```python
from build123d import *

# Parameters (mm, degrees)
SKETCH1_R           = 177.8
BOSS_EXTRUDE1_DEPTH = 12.7
SKETCH2_R           = 12.7
BOSS_EXTRUDE2_DEPTH = 101.6


with BuildPart() as part:
    # Sketch1 → Boss-Extrude1 (new body, symmetric)
    with BuildSketch(Plane(origin=(0, 0, 0), x_dir=(1, 0, 0), z_dir=(0, 1, 0))):
        Circle(SKETCH1_R)
    extrude(amount=BOSS_EXTRUDE1_DEPTH, both=True)

    # Sketch2 → Boss-Extrude2 (add)
    with BuildSketch(Plane(origin=(0, 12.7, 0), x_dir=(1, 0, 0), z_dir=(0, 1, 0))):
        with Locations((0, 88.9)):
            Circle(SKETCH2_R)
        with Locations((0, -88.9)):
            Circle(SKETCH2_R)
        with Locations((88.9, 0)):
            Circle(SKETCH2_R)
        with Locations((-88.9, 0)):
            Circle(SKETCH2_R)
    extrude(amount=BOSS_EXTRUDE2_DEPTH)


solid = part.part
```
Geometry check sheet. Reference: the model listing, model coordinates, mm. A direction names the side the tool comes from. Coordinates: 2 decimals unless noted, no trailing zeros. Loops run counter-clockwise (first coordinate to the right, second up) from the corner with the lowest first, then second, coordinate; pieces in that order, holes last. Notation, with made-up numbers: (39.5, 88) - (84.5, 88) arc R13 ccw to (84.5, 103) - close; hole circle Ø10 at (73.25, -38). An arc over 180 degrees is marked (long way). One line per item, written item: value. Start each with the question number.
(1) Depth check by flat-ended pin: P1, Ø5, axis at x = -99, z = -65, coming from the +Y side; P2, Ø10, axis at y = 79, z = 4, coming from the -X side. Enter the tip coordinate at first touch or a pass-through.
(2) Cross-section at C-C on x = -88.9. Enter the section's corners in (y, z).
(3) Cross-section at B-B on y = 42. Enter the section's corners in (x, z).
(4) Material ranges on line 1 (Y direction, x = -51.5, z = 98.5); line 2 (Z direction, x = 11.5, y = 30.5); line 3 (X direction, y = -0.5, z = -37), recorded low to high. Write a range as [from, to].
(5) Tool access check on faces 4 (the cylindrical face through (169.59, 0.18, -53.41)), 5 (the cylindrical face through (-1.653, 62.789, 76.308)). Record the directions out of +Z, -Z, +X, -X, +Y, -Y that give a thin tool (end or side, any length) a straight path to the whole face; none if there is none.
(6) Cross-section at A-A on z = 0. Enter the section's corners in (x, y), plus the area to 3 significant figures.
(7) Cross-section at D-D on y = 0. Enter the section's corners in (x, z).
(8) Mould release check, pull along Z, two halves, no side actions. Record for faces 1 (the cylindrical face through (101.014, 62.789, -3.815)), 2 (the cylindrical face through (-1.653, 62.789, -101.492)), 3 (the flat face through (0, 114.3, -89)): released by +Z, released by -Z, zero draft, split by the parting line, or undercut.
Results below:
1. P1: stops at y = 12.7
1. P2: stops at x = -101.6
2. outline: (-12.7, -153.98) - (12.7, -153.98) - (12.7, -12.7) - (114.3, -12.7) - (114.3, 12.7) - (12.7, 12.7) - (12.7, 153.98) - (-12.7, 153.98) - close
3. outline: circle Ø25.4 at (-88.9, 0); circle Ø25.4 at (0, -88.9); circle Ø25.4 at (0, 88.9); circle Ø25.4 at (88.9, 0)
4. line 1: y = [-12.7, 12.7]
4. line 2: z = [-94.29, -83.51], [83.51, 94.29]
4. line 3: x = [-173.91, 173.91]
5. face 4: +Y, -Y
5. face 5: +Y
6. outline: (-177.8, -12.7) - (177.8, -12.7) - (177.8, 12.7) - (101.6, 12.7) - (101.6, 114.3) - (76.2, 114.3) - (76.2, 12.7) - (-76.2, 12.7) - (-76.2, 114.3) - (-101.6, 114.3) - (-101.6, 12.7) - (-177.8, 12.7) - close
6. area: 14,200 mm2
7. outline: circle Ø355.6 at (0, 0)
8. face 1: split by the parting line
8. face 2: undercut
8. face 3: zero draft
